from build123d import *

# Parameters (mm, degrees)
F0_R      = 9.525
F1_DEPTH  = 25.4
F3_DEPTH  = 25.401
F4_DEPTH  = 11.0998
F6_DEPTH  = 9.525
F7_R      = 0.75
F8_DEPTH  = 2
F10_DEPTH = 27.401
F11_D     = 0.8
F12_R     = 2
F13_DEPTH = 25


with BuildPart() as f1:
    # F0 (on Front) → F1 (new body)
    with BuildSketch(Plane.XZ):
        Circle(F0_R)
    extrude(amount=F1_DEPTH)

    # F2 (on Front) → F3 (cut, through all)
    with BuildSketch(Plane.XZ):
        with BuildLine():
            ThreePointArc((4.7625, 0), (3.367596, 3.367596), (0, 4.7625))
            ThreePointArc((0, 4.7625), (-3.367596, 3.367596), (-4.7625, 0))
            ThreePointArc((-4.7625, 0), (-3.367596, -3.367596), (0, -4.7625))
            ThreePointArc((0, -4.7625), (3.367596, -3.367596), (4.7625, 0))
        make_face()
    extrude(amount=F3_DEPTH, mode=Mode.SUBTRACT)

    # F2 (on Front) → F4 (cut)
    with BuildSketch(Plane.XZ):
        with BuildLine():
            Line((4.7625, 0), (4.7625, 4.7625))
            Line((4.7625, 4.7625), (0, 4.7625))
            ThreePointArc((0, 4.7625), (3.367596, 3.367596), (4.7625, 0))
        make_face()
        with BuildLine():
            ThreePointArc((-4.7625, 0), (-3.367596, 3.367596), (0, 4.7625))
            Line((0, 4.7625), (-4.7625, 4.7625))
            Line((-4.7625, 4.7625), (-4.7625, 0))
        make_face()
        with BuildLine():
            Line((4.7625, -4.7625), (4.7625, 0))
            ThreePointArc((4.7625, 0), (3.367596, -3.367596), (0, -4.7625))
            Line((0, -4.7625), (4.7625, -4.7625))
        make_face()
        with BuildLine():
            ThreePointArc((0, -4.7625), (-3.367596, -3.367596), (-4.7625, 0))
            Line((-4.7625, 0), (-4.7625, -4.7625))
            Line((-4.7625, -4.7625), (0, -4.7625))
        make_face()
    extrude(amount=F4_DEPTH, mode=Mode.SUBTRACT)

    # F5 (on face) → F6 (cut)
    with BuildSketch(Plane.XZ.offset(25.4)):
        Polygon((7.301568, 0.116642), (3.549769, 6.381665), (-3.751799, 6.265023), (-7.301568, -0.116642), (-3.549769, -6.381665), (3.751799, -6.265023), align=None)
    extrude(amount=-F6_DEPTH, mode=Mode.SUBTRACT)

    # F7 (on face) → F8 (join)
    with BuildSketch(Plane.XZ.offset(25.4)):
        with Locations((6.970895, -3.485664)):
            Circle(F7_R)
    extrude(amount=F8_DEPTH)

    # F9 (on face) → F10 (cut, through all)
    with BuildSketch(Plane.XZ.offset(27.4)):
        Polygon((7.117352, -3.963734), (7.311686, -3.119794), (6.483646, -3.373465), align=None)
    extrude(amount=-F10_DEPTH, mode=Mode.SUBTRACT)

    # F11 (through all)
    with Locations(Plane.XZ.offset(27.4)):
        with Locations((6.970895, -3.485664)):
            Hole(F11_D / 2)

    # F12 (on face) → F13 (cut)
    with BuildSketch(Plane(origin=(-5.425669, 0, -3.249153), x_dir=(0, 1, 0), z_dir=(0.857928, 0, 0.513769))):
        with Locations((-18.914583, 0)):
            Circle(F12_R)
    extrude(amount=-F13_DEPTH, mode=Mode.SUBTRACT)


solid = f1.part
Verification items for the finished model (mm, model axes). A direction names the side the tool comes from. Round coordinates to 2 decimals unless told otherwise and drop trailing zeros. Write each loop counter-clockwise with the first axis right and the second up, starting at its lowest first coordinate (ties: lowest second). Pieces come first, ordered by that corner, then holes.
(1) Access from +Z, -Z, +X, -X, +Y, -Y to the whole of each face (thin tool, end or side, straight path). Record for faces 1 (the flat face through (0, -5, 4.762)), 2 (the flat face through (0, 0, -6)), 3 (the flat face through (5.5, -20.7, -3.12)).
Returned:
face 1: +Y
face 2: +Z, -Z, +X, -X, +Y
face 3: -Y
(2) Section check C-C (y = -21.25). Enter the section's corners in (x, z) (3 decimals), plus the area to 3 significant figures.
Returned:
outline: circle Ø19.05 at (0, 0); hole (-7.302, -0.117) - (-3.55, -6.382) - (3.752, -6.265) - (7.302, 0.117) - (3.55, 6.382) - (-3.752, 6.265) - close; hole (6.484, -3.373) - (6.572, -3.456) arc R0.4 ccw to (7.029, -3.881) - (7.117, -3.964) - (7.144, -3.846) arc R0.4 ccw to (7.285, -3.237) - (7.312, -3.12) - (7.196, -3.155) arc R0.4 ccw to (6.599, -3.338) - close
area: 146 mm2
(3) Section check A-A (y = -2.75). Give the number of separate pieces and of enclosed holes in the cut face, plus the area to 3 significant figures.
Returned:
separate pieces: 1
enclosed holes: 2
area: 194 mm2
(4) Mould release check, pull along X, two halves, no side actions. Record for faces 4 (the flat face through (5.45, -20.7, 3.21)), 5 (the cylindrical face through (9.085, -12.522, 2.861)), 6 (the flat face through (6.2, -25.4, 2.3)): pulls with the +X half, pulls with the -X half, needs draft (parallel to the pull), parting line crosses it, or undercut.
Returned:
face 4: undercut
face 5: parting line crosses it
face 6: needs draft
(5) Section check B-B (x = -2.25). Enter the section's corners in (y, z) (1 decimal).
Returned:
outline: (-25.4, -9.3) - (0, -9.3) - (0, -4.8) - (-11.1, -4.8) - (-11.1, -4.2) - (-15.9, -4.2) - (-15.9, -6.4) - (-25.4, -6.4) - close; (-25.4, 6.3) - (-15.9, 6.3) - (-15.9, 4.2) - (-11.1, 4.2) - (-11.1, 4.8) - (0, 4.8) - (0, 9.3) - (-25.4, 9.3) - close
(6) Material ranges on line 1 (X direction, y = -21, z = -3.5); line 2 (Z direction, x = 8.25, y = -9.5); line 3 (Y direction, x = 2.5, z = -7.25), recorded low to high.
Returned:
line 1: x = -8.86 to -5.28, 5.29 to 6.57, 7.37 to 8.86
line 2: z = -4.76 to 4.76
line 3: y = -25.4 to 0
(7) Depth check by flat-ended pin: pin 1 Ø1 at (x, y) = (6, -14.5) entering from -Z; pin 2 Ø1 at (y, z) = (-13.5, -2.5) entering from +X; pin 3 Ø5 at (y, z) = (-12.5, -5) entering from +X. Enter the tip coordinate at first touch or a pass-through.
Returned:
pin 1: stops at z = -7.78
pin 2: stops at x = 9.31
pin 3: stops at x = 9.19
